Input: part model. Units: mm. Frame: model coordinates. Give positions to 0.01 mm unless a question says otherwise; leave off trailing zeros. Write each loop counter-clockwise with the first axis right and the second up, starting at its lowest first coordinate (ties: lowest second). Pieces come first, ordered by that corner, then holes. Notation, with made-up numbers: (-28.5, 36.25) - (20.5, 36.25) arc R33 cw to (20.5, 74.25) - close; hole circle Ø11 at (69, -30). An arc over 180 degrees is marked (long way). Answer as CSV lines item,"result". Start each with the question number.
from build123d import *

# Parameters (mm, degrees)
BOSS_EXTRUDE1_DEPTH = 12.7
SKETCH6_W           = 114.815330755
SKETCH6_H           = 104.276185761
CUT_EXTRUDE3_DEPTH  = 12.7
SKETCH7_W           = 122.360161844
SKETCH7_H           = 106.085242249
CUT_EXTRUDE4_DEPTH  = 12.7
CUT_EXTRUDE5_DEPTH  = 877.31520365
SKETCH9_W           = 128.341826347
SKETCH9_H           = 668.528804507
CUT_EXTRUDE6_DEPTH  = 877.394501708
SKETCH10_W          = 113.997044676
SKETCH10_H          = 648.207852324
CUT_EXTRUDE7_DEPTH  = 876.98732182
SKETCH12_W          = 87.20410609
SKETCH12_H          = 734.299119323
CUT_EXTRUDE9_DEPTH  = 868.461646496
SKETCH14_W          = 100.100558247
SKETCH14_H          = 114.490742636
CUT_EXTRUDE10_DEPTH = 12.7
SKETCH15_W          = 127.653675673
SKETCH15_H          = 100.172241776
CUT_EXTRUDE11_DEPTH = 861.862470972
SKETCH16_W          = 131.855297217
SKETCH16_H          = 679.360405527
CUT_EXTRUDE12_DEPTH = 877.165513574
SKETCH17_W          = 119.305490094
SKETCH17_H          = 642.509473181
CUT_EXTRUDE13_DEPTH = 877.394501708
SKETCH18_W          = 98.994393467
SKETCH18_H          = 639.457225447
CUT_EXTRUDE14_DEPTH = 877.31520365
SKETCH19_W          = 99.565921338
SKETCH19_H          = 666.000675121
CUT_EXTRUDE15_DEPTH = 877.394501708
SKETCH20_R          = 4.7625
CUT_EXTRUDE16_DEPTH = 508


# Read off the part's stored shape, not the designer's step: Mirror1
with BuildPart() as part:
    # Sketch1 → Boss-Extrude1 (new, symmetric)
    with BuildSketch(Plane.XY):
        Polygon((52.417084438, 236.384308448), (90.152766869, 236.384308448), (90.152766869, 866.253701631), (46.187524325, 799.857212891), align=None)
        Polygon((90.152766869, 866.253701631), (90.152766869, 236.384308448), (127.8884493, 236.384308448), (134.118009413, 799.857212891), align=None)
    extrude(amount=BOSS_EXTRUDE1_DEPTH, both=True)

    # Sketch6 → Cut-Extrude3 (cut)
    with BuildSketch(Plane(origin=(-80.475493735, 53.287826933, 172.016834397), x_dir=(-0.9129832156192912, -0.12073015458483159, -0.3897253876402993), z_dir=(0.4079971176337633, -0.27016025356830164, -0.8720962042082583))):
        with Locations((-159.579476902, 801.401673743)):
            Rectangle(SKETCH6_W, SKETCH6_H)
    extrude(amount=-CUT_EXTRUDE3_DEPTH, mode=Mode.SUBTRACT)

    # Sketch7 → Cut-Extrude4 (cut)
    with BuildSketch(Plane(origin=(110.489450025, 73.161933124, 236.171839964), x_dir=(0.9129832156192915, -0.12073015458482926, -0.3897253876402993), z_dir=(0.4079971176337626, 0.2701602535682969, 0.8720962042082602))):
        with Locations((1.839292518, 801.972236913)):
            Rectangle(SKETCH7_W, SKETCH7_H)
    extrude(amount=CUT_EXTRUDE4_DEPTH, mode=Mode.SUBTRACT)

    # Sketch8 → Cut-Extrude5 (cut, through all)
    with BuildSketch(Plane(origin=(12.74567879, -0.140911784, 37.871408439), x_dir=(0.947764978993365, 0.0011868122313308312, -0.31896729623965236), z_dir=(0.31896950417509595, -0.0035264157067469155, 0.9477584184793911))):
        Polygon((81.673294324, 236.429925956), (128.061632698, 799.851676208), (231.741614255, 799.851676208), (231.741614255, 224.074314905), align=None)
    extrude(amount=CUT_EXTRUDE5_DEPTH, mode=Mode.SUBTRACT)

    # Sketch9 → Cut-Extrude6 (cut, through all)
    with BuildSketch(Plane(origin=(10.329270127, 0, 35.75817846), x_dir=(-0.9607204173379366, 0, 0.27751807096119224), z_dir=(-0.27751807096119224, 0, -0.9607204173379366))):
        with Locations((-110.06191607, 531.852930857)):
            Rectangle(SKETCH9_W, SKETCH9_H)
    extrude(amount=-CUT_EXTRUDE6_DEPTH, mode=Mode.SUBTRACT)

    # Sketch10 → Cut-Extrude7 (cut, through all)
    with BuildSketch(Plane(origin=(6.175448175, 0.216498836, -18.349193008), x_dir=(-0.9477710226369341, 0.0037629901372113698, -0.3189293472776808), z_dir=(0.31895154592781055, 0.011181801925878497, -0.9477050588954087))):
        with Locations((-63.898815232, 515.571273572)):
            Rectangle(SKETCH10_W, SKETCH10_H)
    extrude(amount=-CUT_EXTRUDE7_DEPTH, mode=Mode.SUBTRACT)

    # Sketch12 → Cut-Extrude9 (cut, through all)
    with BuildSketch(Plane(origin=(90.152766869, 0, 0), x_dir=(0, 0, -1), z_dir=(1, 0, 0))):
        with Locations((-8.892958554, 531.759474075)):
            Rectangle(SKETCH12_W, SKETCH12_H)
    extrude(amount=-CUT_EXTRUDE9_DEPTH, mode=Mode.SUBTRACT)

    # Mirror1: part across plane


with BuildPart() as part_1:
    add(part.part)
    add(part.part.mirror(Plane.ZY.offset(-90.152766869)))

    # Sketch14 → Cut-Extrude10 (cut)
    with BuildSketch(Plane(origin=(110.489450025, 73.161933124, -236.171839964), x_dir=(0.9129832156192876, -0.12073015458483696, 0.3897253876403062), z_dir=(-0.40799711763377144, -0.2701602535683071, 0.8720962042082528))):
        with Locations((-13.369077843, 796.553249818)):
            Rectangle(SKETCH14_W, SKETCH14_H)
    extrude(amount=-CUT_EXTRUDE10_DEPTH, mode=Mode.SUBTRACT)

    # Sketch15 → Cut-Extrude11 (cut, through all)
    with BuildSketch(Plane(origin=(-80.475493735, 53.287826933, -172.016834397), x_dir=(-0.9129832156192877, -0.12073015458483585, 0.3897253876403061), z_dir=(-0.4079971176337711, 0.270160253568305, -0.8720962042082536))):
        with Locations((-157.367388135, 783.503693327)):
            Rectangle(SKETCH15_W, SKETCH15_H)
    extrude(amount=CUT_EXTRUDE11_DEPTH, mode=Mode.SUBTRACT)

    # Sketch16 → Cut-Extrude12 (cut, through all)
    with BuildSketch(Plane(origin=(5.598884712, 0.061899319, 16.636042161), x_dir=(0.9477649789933651, -0.0011868122313305589, -0.3189672962396519), z_dir=(0.31896950417509556, 0.0035264157067461093, 0.9477584184793914))):
        with Locations((56.359358162, 528.47269788)):
            Rectangle(SKETCH16_W, SKETCH16_H)
    extrude(amount=-CUT_EXTRUDE12_DEPTH, mode=Mode.SUBTRACT)

    # Sketch17 → Cut-Extrude13 (cut, through all)
    with BuildSketch(Plane(origin=(3.557191293, 0, 12.314391965), x_dir=(0.9607204173379333, 0, -0.27751807096120285), z_dir=(0.27751807096120285, 0, 0.9607204173379335))):
        with Locations((80.7028718, 538.35243952)):
            Rectangle(SKETCH17_W, SKETCH17_H)
    extrude(amount=-CUT_EXTRUDE13_DEPTH, mode=Mode.SUBTRACT)

    # Sketch18 → Cut-Extrude14 (cut, through all)
    with BuildSketch(Plane(origin=(12.74567879, -0.140911784, -37.871408439), x_dir=(-0.9477649789933651, -0.001186812231330454, -0.31896729623965203), z_dir=(0.31896950417509573, -0.0035264157067457975, -0.9477584184793914))):
        with Locations((-106.935938294, 529.421515118)):
            Rectangle(SKETCH18_W, SKETCH18_H)
    extrude(amount=CUT_EXTRUDE14_DEPTH, mode=Mode.SUBTRACT)

    # Sketch19 → Cut-Extrude15 (cut, through all)
    with BuildSketch(Plane(origin=(10.329270127, 0, -35.75817846), x_dir=(0.9607204173379326, 0, 0.2775180709612057), z_dir=(-0.2775180709612056, 0, 0.9607204173379325))):
        with Locations((102.080018676, 535.484996681)):
            Rectangle(SKETCH19_W, SKETCH19_H)
    extrude(amount=-CUT_EXTRUDE15_DEPTH, mode=Mode.SUBTRACT)

    # Sketch20 → Cut-Extrude16 (cut)
    with BuildSketch(Plane.XZ.offset(-236.384308448)):
        with Locations(Location((90.152766869, 0, 0), (0, 0, 270))):
            Circle(SKETCH20_R)
    extrude(amount=-CUT_EXTRUDE16_DEPTH, mode=Mode.SUBTRACT)


solid = part_1.part
1) Cut plane A-A on y = 604.5. Output: boundary loops of the cut face in (x, z) (1 decimal).
2) Cut plane B-B on x = 112.5. Output: boundary loops of the cut face in (y, z).
3) Cut plane C-C on y = 371. Output: boundary loops of the cut face in (x, z) (1 decimal), and give its area (3 significant figures).
4) Contact query for a flat-ended pin moving along its axis: P1, Ø3, axis at x = 122, y = 692, coming from the -Z side. Output: stop coordinate, or through.
5) Material intervals for line 1 (Z direction, x = 90, y = 560); line 2 (Z direction, x = 113, y = 763); line 3 (Z direction, x = 94, y = 511.5), sorted ascending. Write a range as from..to.
Numbers:
1,outline,"(48.3, 0) - (61.4, -4.4) - (90.2, -12.7) - (118.9, -4.4) - (132, 0) - (118.9, 4.4) - (90.2, 12.7) - (61.4, 4.4) - close; hole circle Ø9.5 at (90.2, 0)"
2,outline,"(236.38, -5.18) - (522.79, -6.24) - (812.35, -6.24) - (832.5, 0) - (812.35, 6.24) - (522.79, 6.24) - (236.38, 5.18) - close"
3,outline,"(50.9, 0) - (79.6, -9.7) - (90.2, -12.7) - (100.7, -9.7) - (129.4, 0) - (100.7, 9.7) - (90.2, 12.7) - (79.6, 9.7) - close; hole circle Ø9.5 at (90.2, 0)"
3,area,"954 mm²"
4,P1,"stops at z = -3.93"
5,line 1,"z = -12.66..-4.76, 4.76..12.66"
5,line 2,"z = -6.1..6.1"
5,line 3,"z = -11.59..-2.81, 2.81..11.59"
